```python
from build123d import *

# Parameters (mm, degrees)
F0_W           = 38.1
F0_H           = 50.8
F1_DEPTH       = 25.4
F2_R           = 8.001
F3_DEPTH       = 38.101
F4_R           = 2.9972
F5_DEPTH       = 32.270091028
F6_R           = 9.525
F8_D           = 3.7973
F8_CSINK_D     = 4.318
F8_CSINK_ANGLE = 90
F9_R           = 3.81
F10_DEPTH      = 8.89
F11_R          = 3.81
F12_DEPTH      = 8.89
F14_DEPTH      = 38.1010001
F15_R          = 5.842
F16_DEPTH      = 25.401


with BuildPart() as f1:
    # F0 (on Top) → F1 (new body)
    with BuildSketch(Plane.XY):
        Rectangle(F0_W, F0_H)
    extrude(amount=F1_DEPTH)

    # F2 (on face) → F3 (cut, through all)
    with BuildSketch(Plane.YZ.offset(19.05)):
        with Locations((14.2875, 12.7)):
            Circle(F2_R)
    extrude(amount=-F3_DEPTH, mode=Mode.SUBTRACT)

    # F4 (on face) → F5 (cut, through all)
    with BuildSketch(Plane.XZ.offset(25.4)):
        with Locations((0, 12.7)):
            Circle(F4_R)
    extrude(amount=-F5_DEPTH, mode=Mode.SUBTRACT)

    # F6
    f6_edges = [f1.edges().sort_by_distance(p)[0] for p in [
        (0, 25.4, 25.4),
        (0, 25.4, 0),
    ]]
    fillet(f6_edges, radius=F6_R)

    # F8 (through all)
    with Locations(Plane.XY.offset(25.4)):
        with Locations((-9.525, -1.5875), (-9.525, -20.6375), (9.525, -20.6375), (9.525, -1.5875)):
            CounterSinkHole(F8_D / 2, F8_CSINK_D / 2, counter_sink_angle=F8_CSINK_ANGLE)

    # F9 (on face) → F10 (cut)
    with BuildSketch(Plane.XY.offset(25.4)):
        with Locations((9.525, -1.5875)):
            Circle(F9_R)
        with Locations((9.525, -20.6375)):
            Circle(F9_R)
    extrude(amount=-F10_DEPTH, mode=Mode.SUBTRACT)

    # F11 (on face) → F12 (cut)
    with BuildSketch(Plane(origin=(0, 0, 0), x_dir=(1, 0, 0), z_dir=(0, 0, -1))):
        with Locations((-9.525, 20.6375)):
            Circle(F11_R)
        with Locations((-9.525, 1.5875)):
            Circle(F11_R)
    extrude(amount=-F12_DEPTH, mode=Mode.SUBTRACT)

    # F13 (on face) → F14 (cut, through all)
    with BuildSketch(Plane(origin=(-19.05, 0, 0), x_dir=(0, -1, 0), z_dir=(-1, 0, 0))):
        Polygon((25.4, 22.86), (25.4, 25.4), (-8.89, 25.4), (-6.35, 22.86), align=None)
        Polygon((-8.89, 0), (25.4, 0), (25.4, 2.54), (-6.35, 2.54), align=None)
    extrude(amount=-F14_DEPTH, mode=Mode.SUBTRACT)

    # F15 (on face) → F16 (cut, through all)
    with BuildSketch(Plane.XY.offset(25.4)):
        with Locations((0, 14.2875)):
            Circle(F15_R)
    extrude(amount=-F16_DEPTH, mode=Mode.SUBTRACT)


solid = f1.part
```
Can you work these out from the model? Positions are in its coordinate system, mm. A direction names the side the tool comes from. Give positions to 0.01 mm unless a question says otherwise; leave off trailing zeros. Order: outer loops, then holes, each group sorted by start corner. A loop starts at its lowest first (then second) coordinate and runs counter-clockwise, first axis right, second up. Notation, with made-up numbers: M 82.25,52.25 L 106.25,52.25 A23 cw 106.25,75.25 Z; hole C 51.5,28.25 d9. An arc over 180 degrees is marked long. Write item = value, one per line. Start each with the question number.
Q1. For faces 1 (the cylindrical face through (-0.65, -9.491, 9.774)), 2 (the flat face through (0, -10, 2.54)), 3 (the cylindrical face through (-12.333, -23.212, 5.671)), which set-ups out of +Z, -Z, +X, -X, +Y, -Y let a thin tool reach every point of the face, with its end or its side?
Q2. Suppose I cut it at A-A (z = 14.75). Count the separate pieces of the cut face and the enclosed holes in it, plus the area to 3 significant figures.
Q3. I need wall thicknesses on probe 1 along Y at (x, z) = (-8.5, 18.75); probe 2 along Y at (x, z) = (-11, 3.5); probe 3 along Y at (x, z) = (13, 17.25). Which ranges of each line are inside material? Lowest first, please. Write a range as [from, to].
Q4. We'd pull the mould along X, two halves only. Please class faces 4 (the flat face through (-8, 0, 8.89)), 5 (the flat face through (-0.27, 7.6, 1.29)), 6 (the cylindrical face through (5.72, -1.42, 19.73)), 7 (the flat face through (19.05, 0, 13)): pulls with the +X half, pulls with the -X half, needs draft (parallel to the pull), parting line crosses it, or undercut.
Q5. Will these pins go through, and if not, where does the flat tip stop? pin 1 Ø12 at (x, y) = (-9.52, -1.59) entering from +Z; pin 2 Ø9.5 at (y, z) = (14.29, 12.7) entering from +X; pin 3 Ø10 at (x, y) = (-2, 19.5) entering from -Z; pin 4 Ø5 at (x, z) = (0, 12.7) entering from -Y.
Q6. Suppose I cut it at C-C (y = 10.5). Write out the boundary of the cut face in (x, z).
Check result:
q1.face_1 = -Y
q1.face_2 = -Z, +X, -X, -Y
q1.face_3 = -Z
q2.separate_pieces = 3
q2.enclosed_holes = 4
q2.area = 1,160 mm2
q3.probe_1 = [-25.4, -22.24], [-19.04, -3.19], [0.01, 9.05], [19.52, 24.96]
q3.probe_2 = [-25.4, -24.15], [-17.12, -5.1], [1.93, 23.25]
q3.probe_3 = [-25.4, -22.2], [-19.08, -3.15], [-0.03, 7.71], [20.87, 25.3]
q4.face_4 = undercut
q4.face_5 = needs draft
q4.face_6 = undercut
q4.face_7 = pulls with the +X half
q5.pin_1 = 22.86
q5.pin_2 = through
q5.pin_3 = 0
q5.pin_4 = 21.89
q6.outline = M -19.05,0 L -4.45,0 L -4.45,5.65 L -19.05,5.65 Z; M -19.05,19.75 L -4.45,19.75 L -4.45,25.4 L -19.05,25.4 Z; M 4.45,0 L 19.05,0 L 19.05,5.65 L 4.45,5.65 Z; M 4.45,19.75 L 19.05,19.75 L 19.05,25.4 L 4.45,25.4 Z
